```python
from build123d import *

# Parameters (mm, degrees)
F0_W     = 60
F0_H     = 50
F1_DEPTH = 35
F2_R     = 5
F3_R     = 10
F4_DEPTH = 30
F5_R     = 14.2018831862
F6_DEPTH = 30
F7_R     = 5.0166024016
F8_DEPTH = 13.3


# Not quite as in the source:
# - the program builds the solid bodies; features that only make, move or delete a surface that nothing else refers to are left out


with BuildPart() as f1:
    # F0 (on Top) → F1 (new body)
    with BuildSketch(Plane.XY):
        with Locations((-30, 25)):
            Rectangle(F0_W, F0_H)
    extrude(amount=F1_DEPTH)

    # F2
    f2_edges = [f1.edges().sort_by_distance(p)[0] for p in [
        (-60, 25, 35),
        (-30, 50, 35),
        (-30, 50, 0),
        (-60, 25, 0),
        (-60, 0, 17.5),
        (0, 50, 17.5),
        (-60, 50, 17.5),
        (0, 0, 17.5),
        (0, 25, 0),
        (0, 25, 35),
        (-30, 0, 35),
        (-30, 0, 0),
    ]]
    fillet(f2_edges, radius=F2_R)

    # F3 (on face) → F4 (cut)
    with BuildSketch(Plane.YZ):
        with Locations((25, 17.5)):
            Circle(F3_R)
    extrude(amount=-F4_DEPTH, mode=Mode.SUBTRACT)

    # F5 (on face) → F6 (cut)
    with BuildSketch(Plane.XY.offset(35)):
        with Locations((-30, 25)):
            Circle(F5_R)
    extrude(amount=-F6_DEPTH, mode=Mode.SUBTRACT)

    # F7 (on face) → F8 (cut)
    with BuildSketch(Plane.XZ):
        with Locations((-30, 17.5)):
            Circle(F7_R)
    extrude(amount=-F8_DEPTH, mode=Mode.SUBTRACT)


solid = f1.part
```
Source: CAD feature listing. Evaluate the final solid. Frame: model axes, mm. A direction names the side the tool comes from. Give positions to 0.01 mm unless a question says otherwise; leave off trailing zeros. Write each loop counter-clockwise with the first axis right and the second up, starting at its lowest first coordinate (ties: lowest second). Pieces come first, ordered by that corner, then holes.
1. Pull-direction query (Y, two-part tool) for faces 3 (the face through (-1, 25, 33)), 4 (the face through (-44.19, 25.62, 20.21)), 5 (the face through (-2, 1, 18)), 6 (the face through (-1, 48, 18)); classes: +Y half, -Y half, draft (parallel to the pull), parting line (faces both ways), or undercut.
2. Section query D-D (x = -39). Return the cut outline in (y, z).
3. Access query for faces 1 (the face through (-30, 49, 33)), 2 (the face through (-9.82, 34.54, 20.5)). Directions: +Z, -Z, +X, -X, +Y, -Y. A direction counts if a zero-diameter tool reaches every point of the face in a straight line with its end or side. Return the directions, or none.
4. Section query A-A (z = 17.5). Return the cut outline in (x, y), then the cut area to 3 significant figures.
5. Section query B-B (x = -12.5). Return the cut outline in (y, z), then the cut area to 3 significant figures.
6. Material intervals for line 1 along Y through (x, z) = (-14, 17.5); line 2 along X through (y, z) = (4.75, 17.5); line 3 along Z through (x, y) = (-27, 4.5), sorted ascending.
7. First-contact query: pin 1 (22.5 mm diameter, centred on x = -30, y = 24.5, fed in from +Z). Flat tip, straight axial feed; report the tip coordinate or a pass-through.
8. Section query C-C (y = 25). Return the cut outline in (x, z).
Output values:
1. face 3: draft
1. face 4: undercut
1. face 5: -Y half
1. face 6: +Y half
2. outline: (0, 5) arc R5 ccw to (5, 0) - (45, 0) arc R5 ccw to (50, 5) - (50, 30) arc R5 ccw to (45, 35) - (35.99, 35) - (35.99, 5) - (14.01, 5) - (14.01, 35) - (5, 35) arc R5 ccw to (0, 30) - close
3. face 1: +Z, +X, -X, +Y
3. face 2: +X
4. outline: (-60, 5) arc R5 ccw to (-55, 0) - (-35.02, 0) - (-35.02, 11.71) arc R14.2 cw (long way) to (-19.92, 35) - (0, 35) - (0, 45) arc R5 ccw to (-5, 50) - (-55, 50) arc R5 ccw to (-60, 45) - close; (-24.98, 0) - (-5, 0) arc R5 ccw to (0, 5) - (0, 15) - (-19.92, 15) arc R14.2 cw to (-24.98, 11.71) - close
4. area: 1,890 mm2
5. outline: (0, 5) arc R5 ccw to (5, 0) - (45, 0) arc R5 ccw to (50, 5) - (50, 30) arc R5 ccw to (45, 35) - (5, 35) arc R5 ccw to (0, 30) - close; hole circle Ø20 at (25, 17.5)
5. area: 1,410 mm2
6. line 1: y = 0 to 15, 35 to 50
6. line 2: x = -59.99 to -35.02, -24.98 to -0.01
6. line 3: z = 0.03 to 13.48, 21.52 to 34.97
7. pin 1: stops at z = 5
8. outline: (-60, 5) arc R5 ccw to (-55, 0) - (-5, 0) arc R5 ccw to (0, 5) - (0, 7.5) - (-15.8, 7.5) - (-15.8, 5) - (-44.2, 5) - (-44.2, 35) - (-55, 35) arc R5 ccw to (-60, 30) - close; (-15.8, 27.5) - (0, 27.5) - (0, 30) arc R5 ccw to (-5, 35) - (-15.8, 35) - close
